from build123d import *

# Parameters (mm, degrees)
F2_R     = 5.985152
F3_DEPTH = 25.4
F4_DEPTH = 25.4


with BuildPart() as f1:
    # F0 (on Front) → F1 (revolve)
    with BuildSketch(Plane.XZ):
        with BuildLine():
            Line((0, 22.130426), (0, 19.426251))
            ThreePointArc((0, 19.426251), (19.426251, 0), (0, -19.426251))
            Line((0, -19.426251), (0, -22.130426))
            ThreePointArc((0, -22.130426), (22.130426, 0), (0, 22.130426))
        make_face()
    revolve(axis=Axis((0, 0, 11.065213), (0, 0, 1)))

    # F2 (on Right) → F3 (cut)
    with BuildSketch(Plane.YZ):
        Circle(F2_R)
    extrude(amount=-F3_DEPTH, mode=Mode.SUBTRACT)

    # F2 (on Right) → F4 (cut)
    with BuildSketch(Plane.YZ):
        Circle(F2_R)
    extrude(amount=F4_DEPTH, mode=Mode.SUBTRACT)


solid = f1.part
Could you check a few things on this model? Use its own coordinates, in mm. Give positions to 0.01 mm unless a question says otherwise; leave off trailing zeros. Write each loop counter-clockwise with the first axis right and the second up, starting at its lowest first coordinate (ties: lowest second). Pieces come first, ordered by that corner, then holes. Notation, with made-up numbers: (62.25, 48.25) - (73.25, 48.25) arc R32 ccw to (73.25, 74.25) - close; hole circle Ø3 at (-35, 47.5). An arc over 180 degrees is marked (long way). Use CSV: the item, a comma, the result in double quotes. Start each with the question number.
Item 1: I want a section at C-C, the plane x = -10.5. Please give me the cut outline in (y, z), then the cut area to 3 significant figures.
Item 2: I'm going to push flat-ended pins straight in: pin 1 (4 mm diameter, centred on x = 12, y = 12.5, fed in from -Z); pin 2 (3 mm diameter, centred on y = 3.5, z = 0.5, fed in from -X); pin 3 (4 mm diameter, centred on x = 9.5, z = -12.5, fed in from -Y); pin 4 (12 mm diameter, centred on x = 7.5, z = 11.5, fed in from +Y). Where does each tip first touch, or does it pass through?
Item 3: I want a section at A-A, the plane y = 0. Please give me the cut outline in (x, z).
Item 4: If I drill on line 1 along Z through (x, y) = (-3.5, -14.5); line 2 along Y through (x, z) = (-20.35, 0); line 3 along Z through (x, y) = (-9, -1), over which ranges is the centre line in solid material (lowest first)?
Item 5: I want a section at D-D, the plane z = 8. Please give me the cut outline in (x, y), then the cut area to 3 significant figures.
Findings:
1,outline,"circle Ø38.96 at (0, 0); hole circle Ø32.69 at (0, 0)"
1,area,"353 mm2"
2,pin 1,"stops at z = -15.96"
2,pin 2,"passes through"
2,pin 3,"stops at y = -17.38"
2,pin 4,"stops at y = 20.74"
3,outline,"(-21.31, -5.99) arc R22.13 ccw to (21.31, -5.99) - (18.48, -5.99) arc R19.43 cw to (-18.48, -5.99) - close; (-21.31, 5.99) - (-18.48, 5.99) arc R19.43 cw to (18.48, 5.99) - (21.31, 5.99) arc R22.13 ccw to start"
4,line 1,"z = -16.35 to -12.45, 12.45 to 16.35"
4,line 2,"y = -8.7 to -5.99, 5.99 to 8.7"
4,line 3,"z = -20.19 to -17.19, 17.19 to 20.19"
5,outline,"circle Ø41.27 at (0, 0); hole circle Ø35.41 at (0, 0)"
5,area,"353 mm2"
